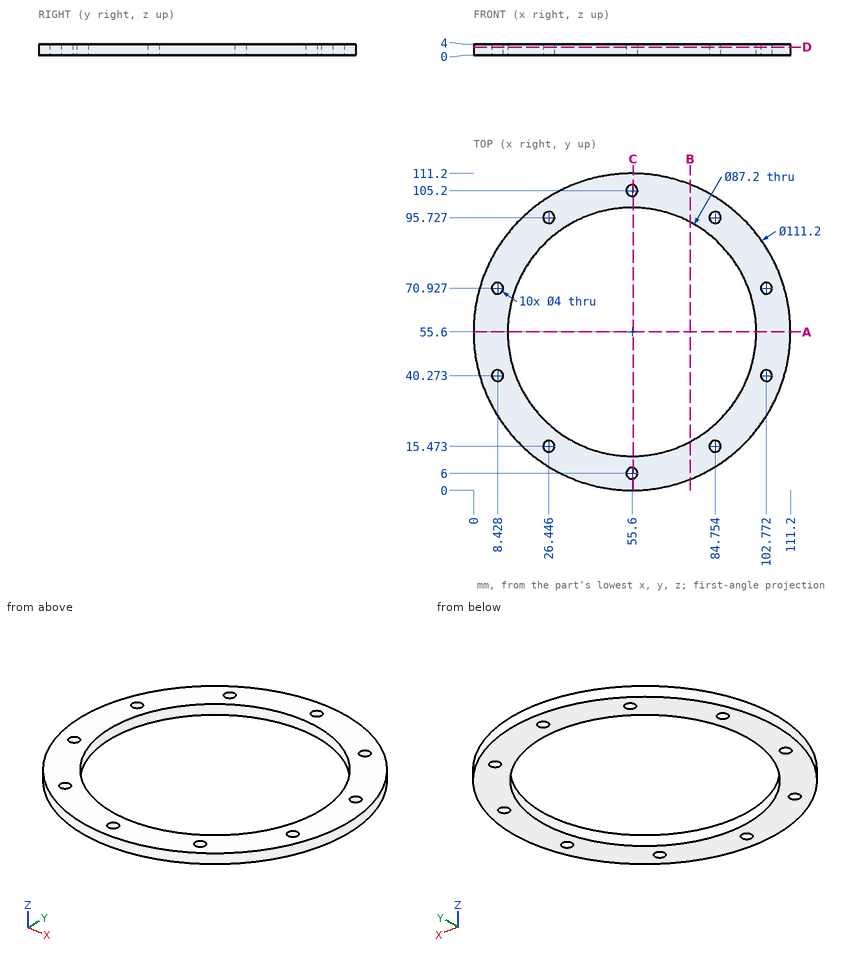
Verification items for this drawing (mm, ordinates from the low corner). Coordinates: 2 decimals unless noted, no trailing zeros. Loops run counter-clockwise (first coordinate to the right, second up) from the corner with the lowest first, then second, coordinate; pieces in that order, holes last. Notation, with made-up numbers: (86, 17.25) -> (107, 17.25) arc R11 ccw to (107, 33.25) -> close; hole circle Ø9 at (66, -4.75). An arc over 180 degrees is marked (long way). Answer in a Markdown table with one row per item. Add a question column.
1. Material ranges on probe 1 along Y at (x, z) = (55.6, 2.7); probe 2 along Y at (x, z) = (53, 2.15); probe 3 along X at (y, z) = (33, 1.7) (1 decimal), recorded low to high. Write a range as [from, to].
2. Section check A-A, the plane y = 55.6. Enter the section's corners in (x, z).
3. Section check C-C, the plane x = 56. Enter the section's corners in (y, z).
4. Section check B-B, the plane x = 76. Enter the section's corners in (y, z).
5. Depth check by flat-ended pin: P1, Ø3.5, axis at x = 84.75, y = 95.73, coming from the -Z side; P2, Ø1.5, axis at x = 27, z = 3, coming from the +Y side; P3, Ø1, axis at y = 71.5, z = 1, coming from the +X side (1 decimal). Enter the tip coordinate at first touch or a pass-through.
6. Section check D-D, the plane z = 2.9. Give the number of separate pieces and of enclosed holes in the cut face, then the cut area to 3 significant figures.
Derived:
| question | item | result |
|---|---|---|
| 1 | probe 1 | y = [0, 4], [8, 12], [99.2, 103.2], [107.2, 111.2] |
| 1 | probe 2 | y = [0.06, 12.08], [99.12, 111.14] |
| 1 | probe 3 | x = [4.8, 18.3], [92.9, 106.4] |
| 2 | outline | (0, 0) -> (12, 0) -> (12, 4) -> (0, 4) -> close; (99.2, 0) -> (111.2, 0) -> (111.2, 4) -> (99.2, 4) -> close |
| 3 | outline | (0, 0) -> (4.04, 0) -> (4.04, 4) -> (0, 4) -> close; (7.96, 0) -> (12, 0) -> (12, 4) -> (7.96, 4) -> close; (99.2, 0) -> (103.24, 0) -> (103.24, 4) -> (99.2, 4) -> close; (107.16, 0) -> (111.2, 0) -> (111.2, 4) -> (107.16, 4) -> close |
| 4 | outline | (3.88, 0) -> (17.07, 0) -> (17.07, 4) -> (3.88, 4) -> close; (94.13, 0) -> (107.32, 0) -> (107.32, 4) -> (94.13, 4) -> close |
| 5 | P1 | passes through |
| 5 | P2 | stops at y = 103.72 |
| 5 | P3 | stops at x = 109 |
| 6 | separate pieces | 1 |
| 6 | enclosed holes | 11 |
| 6 | area | 3,610 mm² |
